The model under review builds one solid part; all positions refer to its coordinate system, in mm. Round coordinates to 2 decimals unless told otherwise and drop trailing zeros. Order: outer loops, then holes, each group sorted by start corner. A loop starts at its lowest first (then second) coordinate and runs counter-clockwise, first axis right, second up.
1) Consider section B-B (z = 1.95). Give the number of separate pieces and of enclosed holes in the cut face, then the cut area to 3 significant figures.
2) Consider section A-A (x = 94.25). Give the boundary of the cut face in (y, z).
3) Mouldability with a two-part tool opening along Y and no side actions: class faces 1 (the face through (-47.727, 10.358, 1.479)), 2 (the face through (-97, 13, 2)), 3 (the face through (-1, 0, 0)) as pulls with the +Y half, pulls with the -Y half, needs draft (parallel to the pull), parting line crosses it, or undercut.
4) To check wall thickness, follow L1, parallel to Y at x = -45, z = 2.1; L2, parallel to Y at x = -63.75, z = 1.3; L3, parallel to X at y = 13, z = 0.95. State the ranges of each line that lie inside material, in increasing order.
Autodesk Inventor part; units mm, degrees
ref_plane "YZ Plane" through (0, 0, 0) normal (1, 0, 0) x (0, 1, 0)
ref_plane "XZ Plane" through (0, 0, 0) normal (0, 1, 0) x (-1, 0, 0)
ref_plane "XY Plane" through (0, 0, 0) normal (0, 0, 1) x (1, 0, 0)
sketch "Sketch1" plane through (0, 0, 0) normal (0, 0, 1) x (1, 0, 0)
  line L0 (-100, -18) -> (100, -18)
  line L1 (100, -18) -> (100, 18)
  line L2 (100, 18) -> (-100, 18)
  line L3 (-100, 18) -> (-100, -18)
  line L4 (-100, -18) -> (100, 18) construction
  line L5 (100, -18) -> (-100, 18) construction
  point P0 (0, 0)
  dimension "d0" = 200
  dimension "d1" = 36
extrude "Extrusion1" add sketch "Sketch1" along normal blind 3
sketch "Sketch2" plane through (0, 0, 3) normal (0, 0, 1) x (1, 0, 0)
  line L0 (-94.25, -13) -> (-63.75, -13)
  line L1 (-63.75, -13) -> (-63.75, 13)
  line L2 (-63.75, 13) -> (-94.25, 13)
  line L3 (-94.25, 13) -> (-94.25, -13)
  line L4 (-94.25, -13) -> (-63.75, 13) construction
  line L5 (-63.75, -13) -> (-94.25, 13) construction
  line L6 (100, 18) -> (-100, 18)
  line L7 (-100, -18) -> (-58, -18)
  line L8 (-58, -18) -> (-58, 18)
  line L9 (-58, 18) -> (-100, 18)
  line L10 (-100, 18) -> (-100, -18)
  line L11 (-100, -18) -> (-58, 18) construction
  line L12 (-58, -18) -> (-100, 18) construction
  line L13 (-100, 18) -> (-100, -18)
  circle A0 centre (-94.25, 13) radius 2.75
  circle A1 centre (-63.75, 13) radius 2.75
  circle A2 centre (-94.25, -13) radius 2.75
  circle A3 centre (-63.75, -13) radius 2.75
  line L14 (63.75, -13) -> (94.25, -13)
  line L15 (94.25, -13) -> (94.25, 13)
  line L16 (94.25, 13) -> (63.75, 13)
  line L17 (63.75, 13) -> (63.75, -13)
  line L18 (63.75, -13) -> (94.25, 13) construction
  line L19 (94.25, -13) -> (63.75, 13) construction
  line L20 (58, -18) -> (100, -18)
  line L21 (100, -18) -> (100, 18)
  line L22 (100, 18) -> (58, 18)
  line L23 (58, 18) -> (58, -18)
  line L24 (58, -18) -> (100, 18) construction
  line L25 (100, -18) -> (58, 18) construction
  circle A4 centre (63.75, 13) radius 2.75
  circle A5 centre (94.25, 13) radius 2.75
  circle A6 centre (63.75, -13) radius 2.75
  circle A7 centre (94.25, -13) radius 2.75
  line L26 (100, -18) -> (100, 18)
  point P0 (0, 0)
  point P1 (-79, 0)
  point P2 (-79, 0)
  point P3 (79, 0)
  point P4 (79, 0)
  dimension "d4" = 30.5
  dimension "d5" = 26
  dimension "d6" = 42
  dimension "d7" = 0
  dimension "d8" = 0
  dimension "d9" = 5.5
  dimension "d10" = 5.5
  dimension "d11" = 5.5
  dimension "d12" = 5.5
  dimension "d13" = 30.5
  dimension "d14" = 26
  dimension "d15" = 42
  dimension "d16" = 0
  dimension "d17" = 5.5
  dimension "d18" = 5.5
  dimension "d19" = 5.5
  dimension "d20" = 5.5
  dimension "d21" = 0
  dimension "d22" = 36
extrude "Extrusion2" cut sketch "Sketch2" against normal blind 3 contours L3 A2 L0 | L0 A2 L3 | A3 L1 L0 | L0 L1 A3 | A0 L2 L3 | L3 L2 A0 | A1 L2 L1 | L1 L2 A1 | L17 A6 L14 | L14 A6 L17 | A7 L15 L14 | L14 L15 A7 | A4 L16 L17 | L17 L16 A4 | A5 L16 L15 | L15 L16 A5
fillet "Fillet1" radius 3 4 edges at (100, 18, 1.5) (100, -18, 1.5) (-100, -18, 1.5) (-100, 18, 1.5)
sketch "Sketch3" plane through (0, 0, 3) normal (0, 0, 1) x (1, 0, 0)
  line L0 (-45, -10) -> (45, -10)
  line L1 (45, -10) -> (45, 10)
  line L2 (45, 10) -> (-45, 10)
  line L3 (-45, 10) -> (-45, -10)
  line L4 (-45, -10) -> (45, 10) construction
  line L5 (45, -10) -> (-45, 10) construction
  point P0 (0, 0)
  dimension "d26" = 90
  dimension "d27" = 20
hole "Hole1" at (-45, 10, 3) at (45, 10, 3) at (45, -10, 3) at (-45, -10, 3) direction (0, 0, -1) diameter 5.5 end through all
properties part number "de ga con truot"
Answer below:
1. separate pieces: 1
1. enclosed holes: 12
1. area: 6,910 mm2
2. outline: (-18, 0) - (-15.75, 0) - (-15.75, 3) - (-18, 3) - close; (-10.25, 0) - (10.25, 0) - (10.25, 3) - (-10.25, 3) - close; (15.75, 0) - (18, 0) - (18, 3) - (15.75, 3) - close
3. face 1: undercut
3. face 2: undercut
3. face 3: needs draft
4. L1: y = -18 to -12.75, -7.25 to 7.25, 12.75 to 18
4. L2: y = -18 to -15.75, -10.25 to 10.25, 15.75 to 18
4. L3: x = -100 to -97, -91.5 to -66.5, -61 to 61, 66.5 to 91.5, 97 to 100
